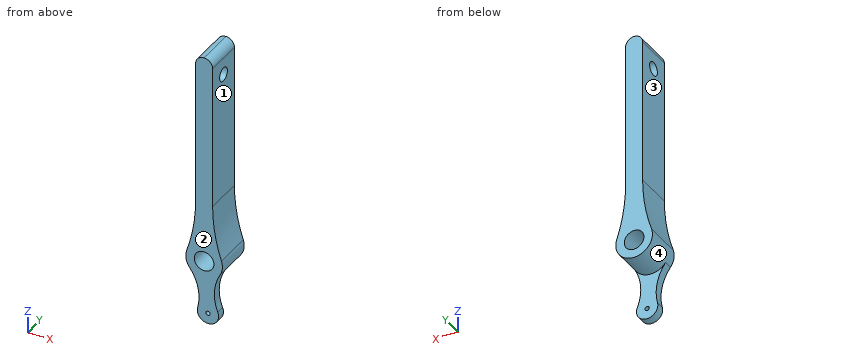
```python
from build123d import *

# Parameters (mm, degrees)
SKETCH1_R           = 14.605
BOSS_EXTRUDE1_DEPTH = 57.15
FILLET1_R           = 254
SKETCH2_R           = 10.16
CUT_EXTRUDE1_DEPTH  = 313.681247479
SKETCH8_R           = 3.175
BOSS_EXTRUDE6_DEPTH = 12.7
SKETCH9_W           = 25.4
SKETCH9_H           = 57.15
BOSS_EXTRUDE7_DEPTH = 12.7
FILLET2_R           = 12.7


with BuildPart() as part:
    # Sketch1 → Boss-Extrude1 (new body)
    with BuildSketch(Plane(origin=(0, 0, 0), x_dir=(1, 0, 0), z_dir=(0, 1, 0))):
        with BuildLine():
            Line((-12.7, -24.171740215), (-12.7, -304.8))
            Line((-12.7, -304.8), (12.7, -304.8))
            Line((12.7, -304.8), (12.7, -24.171740215))
            ThreePointArc((12.7, -24.171740215), (0, 27.305), (-12.7, -24.171740215))
        make_face()
        with Locations(Location((0, 0, 0), (0, 0, 270))):
            Circle(SKETCH1_R, mode=Mode.SUBTRACT)
    extrude(amount=BOSS_EXTRUDE1_DEPTH)

    # Fillet1
    fillet1_edges = [part.edges().sort_by_distance(p)[0] for p in [
        (12.7, 28.575, 24.171740215),
        (-12.7, 28.575, 24.171740215),
    ]]
    fillet(fillet1_edges, radius=FILLET1_R)

    # Sketch2 → Cut-Extrude1 (cut, through all)
    with BuildSketch(Plane.ZY.offset(12.7)):
        with Locations((279.4, 28.575)):
            Circle(SKETCH2_R)
    extrude(amount=-CUT_EXTRUDE1_DEPTH, mode=Mode.SUBTRACT)

    # Sketch8 → Boss-Extrude6 (add)
    with BuildSketch(Plane(origin=(0, 0, 0), x_dir=(1, 0, 0), z_dir=(0, 1, 0))):
        with BuildLine():
            ThreePointArc((20.48678387, 73.276843268), (6.952035658, 95.123295408), (-9.615200393, 75.476830843))
            ThreePointArc((-9.615200393, 75.476830843), (-9.004649416, 44.610856641), (-21.758468792, 16.496425698))
            ThreePointArc((-21.758468792, 16.496425698), (1.990263204, 27.232368193), (23.925719089, 13.157621026))
            ThreePointArc((23.925719089, 13.157621026), (15.395044016, 42.827617971), (20.48678387, 73.276843268))
        make_face()
        with Locations(Location((5.794905888, 79.290523203, 0), (0, 0, 270))):
            Circle(SKETCH8_R, mode=Mode.SUBTRACT)
    extrude(amount=BOSS_EXTRUDE6_DEPTH)

    # Sketch9 → Boss-Extrude7 (add)
    with BuildSketch(Plane.XY.offset(304.8)):
        with Locations((0, 28.575)):
            Rectangle(SKETCH9_W, SKETCH9_H)
    extrude(amount=BOSS_EXTRUDE7_DEPTH)

    # Fillet2
    fillet2_edges = [part.edges().sort_by_distance(p)[0] for p in [
        (-12.7, 28.575, 317.5),
        (12.7, 28.575, 317.5),
    ]]
    fillet(fillet2_edges, radius=FILLET2_R - 0.0001)  # a hair under: the kernel refuses the full size


solid = part.part
```
The listing builds one solid part. Answer for the finished solid, in the listing's coordinates (mm). Face numbers are marked on the shaded views. A direction names the side the tool comes from. Give positions to 0.01 mm unless a question says otherwise; leave off trailing zeros. Order: outer loops, then holes, each group sorted by start corner. A loop starts at its lowest first (then second) coordinate and runs counter-clockwise, first axis right, second up.
Item 1: The part is cut by section C-C, the plane z = 279.4. Give the vertices of the cut face in (x, y) (3 decimals), and give its area (3 significant figures).
From the geometry:
outline: (-12.7, 0) - (12.7, 0) - (12.7, 18.415) - (-12.7, 18.415) - close; (-12.7, 38.735) - (12.7, 38.735) - (12.7, 57.15) - (-12.7, 57.15) - close
area: 935 mm2
Item 2: Which of the six approach directions +Z, -Z, +X, -X, +Y, -Y give full straight-line access (tool end or side, diameter ignored) to the marked faces 1, 2, 3 and 4?
From the geometry:
face 1: +Z, +X, +Y, -Y
face 2: +Z, -Z, +X, -X, -Y
face 3: +Z, -X, +Y, -Y
face 4: +Y
Item 3: Given pin 1 Ø10 at (y, z) = (21, -10.5) entering from +X; pin 2 Ø10 at (x, y) = (5.5, 16.5) entering from +Z; pin 3 Ø5 at (x, z) = (5.79, -79.29) entering from +Y; pin 4 Ø1 at (y, z) = (25, 1) entering from +X, each flat-ended and moving along its own axis, determine where each tip first touches the part or whether it passes through.
From the geometry:
pin 1: stops at x = 26.75
pin 2: stops at z = 317.49
pin 3: passes through
pin 4: stops at x = 27.3
Item 4: The part is cut by section B-B, the plane y = 9. Count the separate pieces of the cut face and the enclosed holes in it, and give its area (3 significant figures).
From the geometry:
separate pieces: 1
enclosed holes: 2
area: 11,300 mm2
Item 5: The part is cut by section D-D, the plane z = 98. Give the vertices of the cut face in (x, y).
From the geometry:
outline: (-12.7, 0) - (12.7, 0) - (12.7, 57.15) - (-12.7, 57.15) - close
Item 6: The part is cut by section A-A, the plane z = 0. Give the vertices of the cut face in (x, y) (3 decimals).
From the geometry:
outline: (-27.305, 0) - (-14.605, 0) - (-14.605, 57.15) - (-27.305, 57.15) - close; (14.605, 0) - (27.305, 0) - (27.305, 57.15) - (14.605, 57.15) - close
Item 7: Find the intervals of material crossed by probe 1 along X at (y, z) = (37, 1.5); probe 2 along Z at (x, y) = (10, 22); probe 3 along Y at (x, z) = (-1, 279.4) (3 decimals), in increasing order.
From the geometry:
probe 1: x = -27.26 to -14.53, 14.53 to 27.26
probe 2: z = -25.41 to -10.64, 10.64 to 271.65, 287.15 to 312.63
probe 3: y = 0 to 18.415, 38.735 to 57.15
